Verification items for the finished model (mm, model axes). Face numbers are marked on the shaded views. Coordinates: 2 decimals unless noted, no trailing zeros. Order: outer loops, then holes, each group sorted by start corner. A loop starts at its lowest first (then second) coordinate and runs counter-clockwise, first axis right, second up. Notation, with made-up numbers: M -11,-13 L 17,-13 A17 cw 17,-8 Z; hole C 68.5,-7 d11. An arc over 180 degrees is marked long. Return JSON: item names as keys, results as strings.
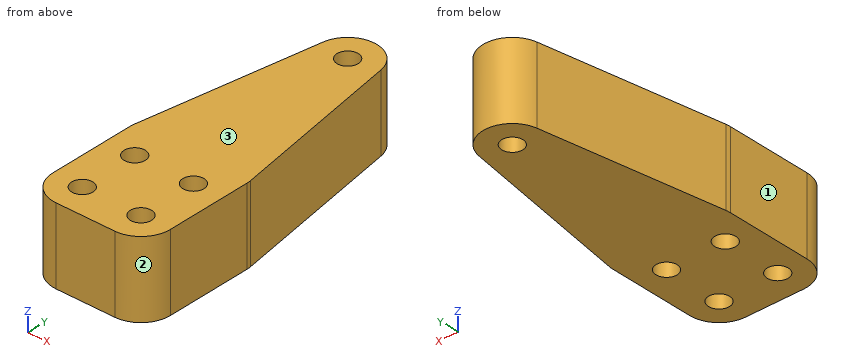
```python
from build123d import *

# Parameters (mm, degrees)
SKETCH1_R           = 2.286
BOSS_EXTRUDE1_DEPTH = 16.51
FILLET1_R           = 6.35


with BuildPart() as part:
    # Sketch1 → Boss-Extrude1 (new body)
    with BuildSketch(Plane.XY):
        with BuildLine():
            Line((-12.7, 12.7), (-6.265860593, 51.830286864))
            ThreePointArc((-6.265860593, 51.830286864), (0, 57.15), (6.265860593, 51.830286864))
            Line((6.265860593, 51.830286864), (12.7, 12.7))
            Line((12.7, 12.7), (12.7, -12.7))
            Line((12.7, -12.7), (-12.7, -12.7))
            Line((-12.7, -12.7), (-12.7, 12.7))
        make_face()
        with Locations((-6.35, -6.35)):
            Circle(SKETCH1_R, mode=Mode.SUBTRACT)
        with Locations((0, 50.8)):
            Circle(SKETCH1_R, mode=Mode.SUBTRACT)
        with Locations((6.35, -6.35)):
            Circle(SKETCH1_R, mode=Mode.SUBTRACT)
        with Locations((6.35, 6.35)):
            Circle(SKETCH1_R, mode=Mode.SUBTRACT)
        with Locations((-6.35, 6.35)):
            Circle(SKETCH1_R, mode=Mode.SUBTRACT)
    extrude(amount=BOSS_EXTRUDE1_DEPTH)

    # Fillet1
    fillet1_edges = [part.edges().sort_by_distance(p)[0] for p in [
        (-12.7, 12.7, 8.255),
        (12.7, 12.7, 8.255),
        (12.7, -12.7, 8.255),
        (-12.7, -12.7, 8.255),
    ]]
    fillet(fillet1_edges, radius=FILLET1_R)


solid = part.part
```
Q1. Cross-section at D-D, the plane y = 50.8. Record the boundary of the cut face in (x, z).
Values:
{"outline": "M -6.44,0 L -2.29,0 L -2.29,16.51 L -6.44,16.51 Z; M 2.29,0 L 6.44,0 L 6.44,16.51 L 2.29,16.51 Z"}
Q2. Go/stop test with flat-tipped pins: pin 1 (1.5 mm diameter, centred on y = 31.5, z = 12, fed in from -X); pin 2 (6 mm diameter, centred on y = 42, z = 9, fed in from -X); pin 3 (8 mm diameter, centred on y = 43, z = 6, fed in from +X). Record where each tip stops, or that it passes through.
Values:
{"pin 1": "x = -9.73", "pin 2": "x = -8.38", "pin 3": "x = 8.38"}
Q3. Draft check along X on the marked faces 1, 2 and 3. Enter one of: pulls with the +X half, pulls with the -X half, needs draft (parallel to the pull), parting line crosses it, or undercut.
Values:
{"face 1": "pulls with the -X half", "face 2": "pulls with the +X half", "face 3": "needs draft"}
Q4. Cross-section at B-B, the plane y = 6.35. Record the boundary of the cut face in (x, z), and give its area (3 significant figures).
Values:
{"outline": "M -12.7,0 L -8.64,0 L -8.64,16.51 L -12.7,16.51 Z; M -4.06,0 L 4.06,0 L 4.06,16.51 L -4.06,16.51 Z; M 8.64,0 L 12.7,0 L 12.7,16.51 L 8.64,16.51 Z", "area": "268 mm^2"}
Q5. Material ranges on line 1 along Y through (x, z) = (5.5, 8); line 2 along Y through (x, z) = (-4.25, 15.5); line 3 along Y through (x, z) = (0.25, 10), recorded low to high.
Values:
{"line 1": "-12.7 to -8.47, -4.23 to 4.23, 8.47 to 53.97", "line 2": "-12.7 to -7.25, -5.45 to 5.45, 7.25 to 55.52", "line 3": "-12.7 to 48.53, 53.07 to 57.15"}
Q6. Cross-section at A-A, the plane x = 0. Record the boundary of the cut face in (y, z).
Values:
{"outline": "M -12.7,0 L 48.51,0 L 48.51,16.51 L -12.7,16.51 Z; M 53.09,0 L 57.15,0 L 57.15,16.51 L 53.09,16.51 Z"}
Q7. Cross-section at C-C, the plane z = 15. Record the boundary of the cut face in (x, y).
Values:
{"outline": "M -12.7,-6.35 A6.35 ccw -6.35,-12.7 L 6.35,-12.7 A6.35 ccw 12.7,-6.35 L 12.7,12.18 A6.35 ccw 12.62,13.21 L 6.27,51.83 A6.35 ccw -6.27,51.83 L -12.62,13.21 A6.35 ccw -12.7,12.18 Z; hole C -6.35,-6.35 d4.57; hole C -6.35,6.35 d4.57; hole C 0,50.8 d4.57; hole C 6.35,-6.35 d4.57; hole C 6.35,6.35 d4.57"}
